from build123d import *

# Parameters (mm, degrees)
F0_R        = 0.9128432721
F0_R_2      = 1.2216898107
F0_R_3      = 1.8377143243
F0_R_4      = 1.1282865395
F0_R_5      = 1.3035270966
F0_R_6      = 0.9702753
F0_R_7      = 2.5484542397
F0_R_8      = 7.7130109431
F1_DEPTH    = 19.05
F2_DEPTH    = 48.26
F4_D        = 5.08
F4_DEPTH    = 12.7
F4_TIP      = 1.5261859723
F5_T1_DEPTH = 40.8239460826
F5_T3_DEPTH = 40.1487670183


# Not quite as in the source:
# - a fillet or chamfer that OpenCascade refuses, or shapes differently, is made with other operations: its cross-section is extruded or revolved along the edge and cut away or added


with BuildPart() as f1:
    # F0 (on Top) → F1 (new body)
    with BuildSketch(Plane.XY):
        with BuildLine():
            Line((-46.1318939924, 34.7651951015), (-46.1318939924, 64.978521944))
            ThreePointArc((-46.1318939924, 64.978521944), (-83.7196043441, 27.3908115923), (-46.1318939924, -10.1968987593))
            Line((-46.1318939924, -10.1968987593), (-46.1318939924, 0.4695183748))
            ThreePointArc((-46.1318939924, 0.4695183748), (-58.2504121537, 4.3055568595), (-65.9541934729, 14.4162159413))
            Line((-65.9541934729, 14.4162159413), (-46.1318939924, 14.4162159413))
            Line((-46.1318939924, 14.4162159413), (-46.1318939924, 20.0164280832))
            Line((-46.1318939924, 20.0164280832), (-53.8438670337, 20.0164280832))
            Line((-53.8438670337, 20.0164280832), (-53.8438670337, 34.7651951015))
            Line((-53.8438670337, 34.7651951015), (-46.1318939924, 34.7651951015))
        make_face()
        with Locations((-69.6755722165, 20.9292713553)):
            Circle(F0_R, mode=Mode.SUBTRACT)
        with Locations((-65.8872798085, 20.9292713553)):
            Circle(F0_R, mode=Mode.SUBTRACT)
        with Locations((-70.7362964749, 23.2022479177)):
            Circle(F0_R_2, mode=Mode.SUBTRACT)
        with Locations((-73.3180493116, 25.5887825042)):
            Circle(F0_R_3, mode=Mode.SUBTRACT)
        with Locations((-67.4026012421, 22.7476526052)):
            Circle(F0_R_4, mode=Mode.SUBTRACT)
        with Locations((-62.856644392, 20.4746760428)):
            Circle(F0_R_5, mode=Mode.SUBTRACT)
        with Locations((-61.4928565919, 24.5660338551)):
            Circle(F0_R_6, mode=Mode.SUBTRACT)
        with Locations((-66.1099404097, 28.1116217375)):
            Circle(F0_R_7, mode=Mode.SUBTRACT)
        with Locations((-63.0709454417, 41.807025671)):
            Circle(F0_R_8, mode=Mode.SUBTRACT)
        with BuildLine():
            ThreePointArc((-46.1318939924, -10.1968987593), (-19.5533691135, 0.8122867134), (-8.5441836408, 27.3908115923))
            ThreePointArc((-8.5441836408, 27.3908115923), (-19.5533691135, 53.9693364713), (-46.1318939924, 64.978521944))
            Line((-46.1318939924, 64.978521944), (-46.1318939924, 34.7651951015))
            Line((-46.1318939924, 34.7651951015), (-38.4199209511, 34.7651951015))
            Line((-38.4199209511, 34.7651951015), (-38.4199209511, 20.0164280832))
            Line((-38.4199209511, 20.0164280832), (-46.1318939924, 20.0164280832))
            Line((-46.1318939924, 20.0164280832), (-46.1318939924, 14.4162159413))
            Line((-46.1318939924, 14.4162159413), (-26.309594512, 14.4162159413))
            ThreePointArc((-26.309594512, 14.4162159413), (-34.0133758311, 4.3055568595), (-46.1318939924, 0.4695183748))
            Line((-46.1318939924, 0.4695183748), (-46.1318939924, -10.1968987593))
        make_face()
        with Locations((-29.4071435928, 20.4746760428)):
            Circle(F0_R_5, mode=Mode.SUBTRACT)
        with Locations((-30.7709313929, 24.5660338551)):
            Circle(F0_R_6, mode=Mode.SUBTRACT)
        with Locations((-26.3765081763, 20.9292713553)):
            Circle(F0_R, mode=Mode.SUBTRACT)
        with Locations((-22.5882157683, 20.9292713553)):
            Circle(F0_R, mode=Mode.SUBTRACT)
        with Locations((-24.8611867428, 22.7476526052)):
            Circle(F0_R_4, mode=Mode.SUBTRACT)
        with Locations((-21.5274915099, 23.2022479177)):
            Circle(F0_R_2, mode=Mode.SUBTRACT)
        with Locations((-18.9457386732, 25.5887825042)):
            Circle(F0_R_3, mode=Mode.SUBTRACT)
        with Locations((-29.1928425431, 41.807025671)):
            Circle(F0_R_8, mode=Mode.SUBTRACT)
        with Locations((-26.1538475752, 28.1116217375)):
            Circle(F0_R_7, mode=Mode.SUBTRACT)
    extrude(amount=F1_DEPTH)

    # F0 (on Top) → F2 (join)
    with BuildSketch(Plane.XY):
        Polygon((-38.4199209511, 34.7651951015), (-46.1318939924, 34.7651951015), (-46.1318939924, 27.3908115923), (-46.1318939924, 20.0164280832), (-38.4199209511, 20.0164280832), align=None)
        Polygon((-46.1318939924, 27.3908115923), (-46.1318939924, 34.7651951015), (-53.8438670337, 34.7651951015), (-53.8438670337, 20.0164280832), (-46.1318939924, 20.0164280832), align=None)
    extrude(amount=F2_DEPTH)

    # F4
    with Locations(Plane.XZ.offset(-20.0164280832)):
        with Locations((-49.9697290361, 43.8477247953), (-43.5725338757, 43.5774177313)):
            Hole(F4_D / 2, depth=F4_DEPTH)
            with Locations((0, 0, -(F4_DEPTH + F4_TIP / 2))):  # 118° drill point
                Cone(0, F4_D / 2, F4_TIP, mode=Mode.SUBTRACT)

    # F5: fillet of radius 5.08 on 4 edges, made by hand

    # F5_s2 → F5_t1 (cut)
    with BuildSketch(Plane.YZ.offset(-66.5438670337)):
        with BuildLine():
            ThreePointArc((34.7651951015, 43.18), (33.2772975499, 46.7721024484), (29.6851951015, 48.26))
            Line((29.6851951015, 48.26), (34.7651951015, 48.26))
            Line((34.7651951015, 48.26), (34.7651951015, 43.18))
        make_face()
        with BuildLine():
            ThreePointArc((20.0164280832, 43.18), (21.5043256348, 46.7721024484), (25.0964280832, 48.26))
            Line((25.0964280832, 48.26), (20.0164280832, 48.26))
            Line((20.0164280832, 48.26), (20.0164280832, 43.18))
        make_face()
    extrude(amount=F5_T1_DEPTH, mode=Mode.SUBTRACT)

    # F5_s4 → F5_t3 (cut)
    with BuildSketch(Plane.XZ.offset(-47.4651951015)):
        with BuildLine():
            ThreePointArc((-53.8438670337, 43.18), (-52.3559694821, 46.7721024484), (-48.7638670337, 48.26))
            Line((-48.7638670337, 48.26), (-53.8438670337, 48.26))
            Line((-53.8438670337, 48.26), (-53.8438670337, 43.18))
        make_face()
        with BuildLine():
            ThreePointArc((-38.4199209511, 43.18), (-39.9078185027, 46.7721024484), (-43.4999209511, 48.26))
            Line((-43.4999209511, 48.26), (-38.4199209511, 48.26))
            Line((-38.4199209511, 48.26), (-38.4199209511, 43.18))
        make_face()
    extrude(amount=F5_T3_DEPTH, mode=Mode.SUBTRACT)


solid = f1.part
Read the model definition and answer for the solid it produces. Units are mm, in the model's axes. A direction names the side the tool comes from. Round coordinates to 2 decimals unless told otherwise and drop trailing zeros. Write each loop counter-clockwise with the first axis right and the second up, starting at its lowest first coordinate (ties: lowest second). Pieces come first, ordered by that corner, then holes.
1. The part is cut by section C-C, the plane z = 17. State how many separate pieces and enclosed holes the cut face has, then the cut area to 3 significant figures.
2. The part is cut by section D-D, the plane y = 45.5. Determine the outline of the cut face in (x, z), then the cut area to 3 significant figures.
3. The part is cut by section A-A, the plane y = 5. Determine the outline of the cut face in (x, z), then the cut area to 3 significant figures.
4. Determine the mould class of faces 1 (the face through (-50.07, 33.98, 43.42)), 2 (the face through (-46.24, 33.878, 46.048)), 3 (the face through (-17.25, 24.88, 9.39)) for opening direction Z: pulls with the +Z half, pulls with the -Z half, needs draft (parallel to the pull), parting line crosses it, or undercut.
5. Which of the six approach directions +Z, -Z, +X, -X, +Y, -Y give full straight-line access (tool end or side, diameter ignored) to faces 4 (the face through (-49.419, 26.455, 41.368)), 5 (the face through (-46, 14.416, 9)), 6 (the face through (-46, 20.016, 31)), 7 (the face through (-47, 28, 0))?
6. Straight lines are drawn through the part: L1, parallel to X at y = 19.5, z = 7; L2, parallel to X at y = 45, z = 4; L3, parallel to Z at x = -40.5, y = 14.5. For each, find the intervals that lie inside material, in ascending order.
7. Given pin 1 Ø2 at (x, z) = (-38, 40) entering from +Y; pin 2 Ø22.5 at (x, y) = (-31.5, 15) entering from +Z; pin 3 Ø2 at (x, y) = (-59.5, 33.5) entering from +Z, each flat-ended and moving along its own axis, determine where each tip first touches the part or whether it passes through.
8. The part is cut by section B-B, the plane x = -19. Determine the outline of the cut face in (y, z), then the cut area to 3 significant figures.
Values:
1. separate pieces: 1
1. enclosed holes: 19
1. area: 3,560 mm2
2. outline: (-79.07, 0) - (-69.84, 0) - (-69.84, 19.05) - (-79.07, 19.05) - close; (-56.3, 0) - (-35.96, 0) - (-35.96, 19.05) - (-56.3, 19.05) - close; (-22.42, 0) - (-13.19, 0) - (-13.19, 19.05) - (-22.42, 19.05) - close
2. area: 739 mm2
3. outline: (-76.32, 0) - (-59.18, 0) - (-59.18, 19.05) - (-76.32, 19.05) - close; (-33.08, 0) - (-15.94, 0) - (-15.94, 19.05) - (-33.08, 19.05) - close
3. area: 653 mm2
4. face 1: undercut
4. face 2: pulls with the +Z half
4. face 3: needs draft
5. face 4: -Y
5. face 5: +Z, -Z
5. face 6: +Z, +X, -X, -Y
5. face 7: -Z, +X, -X, +Y, -Y
6. L1: x = -82.88 to -63.72, -61.99 to -30.27, -28.54 to -9.38
6. L2: x = -79.34 to -70.09, -56.05 to -36.21, -22.17 to -12.92
6. L3: z = 0 to 19.05
7. pin 1: stops at y = 34.77
7. pin 2: stops at z = 47.17
7. pin 3: stops at z = 19.05
8. outline: (1.38, 0) - (23.75, 0) - (23.75, 19.05) - (1.38, 19.05) - close; (27.43, 0) - (53.4, 0) - (53.4, 19.05) - (27.43, 19.05) - close
8. area: 921 mm2
